from build123d import *

# Parameters (mm, degrees)
BASPROSKE_W         = 16
BASPROSKE_H         = 18
TOOTHCUT_DEPTH      = 31.066592757
TEETHCUTS_COUNT     = 16
TEETHCUTS_ANGLE     = 337.5
HUBNEAONESKE_R      = 7.5
HUBNEARONE_DEPTH    = 22.0000508
BORSKE_R            = 5
BORE_DEPTH          = 38.0000508
CUT_EXTRUDE1_START  = -10
SKETCH3_R           = 7.5
CUT_EXTRUDE1_DEPTH  = 10
BOSS_EXTRUDE1_START = -10
SKETCH4_R           = 7.5
BOSS_EXTRUDE1_DEPTH = 10
SKETCH5_R           = 5
BOSS_EXTRUDE2_DEPTH = 10


with BuildPart() as part:
    # BasProSke → Base-Revolve (revolve)
    with BuildSketch(Plane(origin=(0, 0, 0), x_dir=(1, 0, 0), z_dir=(0, 1, 0)), mode=Mode.PRIVATE) as base_revolve_sk:
        with Locations((8, 9)):
            Rectangle(BASPROSKE_W, BASPROSKE_H)
    revolve(base_revolve_sk.sketch.rotate(Axis((-10, 0, 0), (1, 0, 0)), 180), axis=Axis((-10, 0, 0), (1, 0, 0)))

    # TooCutSke → ToothCut (cut, through all)
    with BuildSketch(Plane(origin=(0, 0, 0), x_dir=(0, 0, -1), z_dir=(1, 0, 0))):
        with BuildLine():
            ThreePointArc((1.03434411, 13.459313997), (0, 13.499), (-1.03434411, 13.459313997))
            ThreePointArc((-1.03434411, 13.459313997), (-1.635143665, 15.806872195), (-3.065655864, 17.762792553))
            ThreePointArc((-3.065655864, 17.762792553), (0, 18.0254), (3.065655864, 17.762792553))
            ThreePointArc((3.065655864, 17.762792553), (1.635143665, 15.806872195), (1.03434411, 13.459313997))
        make_face()
    toothcut = extrude(amount=TOOTHCUT_DEPTH, mode=Mode.SUBTRACT)

    # TeethCuts: ToothCut ×16 about axis
    teethcuts_axis = Axis((-10, 0, 0), (1, 0, 0))
    for i in range(1, TEETHCUTS_COUNT):
        add(toothcut.rotate(teethcuts_axis, i * TEETHCUTS_ANGLE / (TEETHCUTS_COUNT - 1)), mode=Mode.SUBTRACT)

    # HubNeaOneSke → HubNearOne (add)
    with BuildSketch(Plane.ZY):
        with Locations(Location((0, 0, 0), (0, 0, 180))):
            Circle(HUBNEAONESKE_R)
    extrude(amount=HUBNEARONE_DEPTH)

    # BorSke → Bore (cut, symmetric)
    with BuildSketch(Plane(origin=(0, 0, 0), x_dir=(0, 0, -1), z_dir=(1, 0, 0))):
        with Locations(Location((0, 0, 0), (0, 0, 180))):
            Circle(BORSKE_R)
    extrude(amount=BORE_DEPTH, both=True, mode=Mode.SUBTRACT)

    # Sketch3 → Cut-Extrude1 (cut)
    with BuildSketch(Plane.ZY.offset(22.0000508).offset(CUT_EXTRUDE1_START)):
        with Locations(Location((0, 0, 0), (0, 0, 180))):
            Circle(SKETCH3_R)
    extrude(amount=CUT_EXTRUDE1_DEPTH, mode=Mode.SUBTRACT)

    # Sketch4 → Boss-Extrude1 (add)
    with BuildSketch(Plane.ZY.offset(12.0000508).offset(BOSS_EXTRUDE1_START)):
        with Locations(Location((0, 0, 0), (0, 0, 180))):
            Circle(SKETCH4_R)
    extrude(amount=BOSS_EXTRUDE1_DEPTH)

    # Sketch5 → Boss-Extrude2 (add)
    with BuildSketch(Plane.ZY.offset(12.0000508)):
        Circle(SKETCH5_R)
    extrude(amount=BOSS_EXTRUDE2_DEPTH)


solid = part.part
Source: CAD feature listing. Evaluate the final solid. Frame: model axes, mm. A direction names the side the tool comes from. Give positions to 0.01 mm unless a question says otherwise; leave off trailing zeros. Write each loop counter-clockwise with the first axis right and the second up, starting at its lowest first coordinate (ties: lowest second). Pieces come first, ordered by that corner, then holes. Notation, with made-up numbers: M 85,73 L 129,73 A19 cw 129,98 Z; hole C 22.5,65 d1. An arc over 180 degrees is marked long. Answer as a JSON object with one key per item and string values.
Q1. Ray query, line 1 along X through (y, z) = (15.5, 2); line 2 along X through (y, z) = (7, -2); line 3 along Y through (x, z) = (6.5, -1). Return the intervals inside material, ascending.
Geometry check:
{"line 1": "x = 0 to 16", "line 2": "x = -12 to 16", "line 3": "y = -13.46 to -4.9, 4.9 to 13.46"}
Q2. Access query for faces 4 (the face through (7.888, 1.614, -15.762)), 5 (the face through (7.89, 15.82, -1.64)), 6 (the face through (7.89, 9.56, 9.53)). Directions: +Z, -Z, +X, -X, +Y, -Y. A direction counts if a zero-diameter tool reaches every point of the face in a straight line with its end or side. Return the directions, or none.
Geometry check:
{"face 4": "-Z, +X, -X", "face 5": "+X, -X, +Y", "face 6": "+X, -X"}
Q3. Contact query for flat-ended pins moving along their axis: P1, Ø5, axis at x = 1.5, z = 12.5, coming from the -Y side; P2, Ø10, axis at x = -5.5, z = -11, coming from the -Y side; P3, Ø2, axis at x = -0.5, y = 5.5, coming from the +Z side. Output: stop coordinate, or through.
Geometry check:
{"P1": "stops at y = -14.97", "P2": "stops at y = -4.5", "P3": "stops at z = 12.68"}
Q4. Cut plane C-C, the plane x = -5. Return the cut outline in (y, z).
Geometry check:
{"outline": "C 0,0 d15"}
Q5. Mould query, pull axis Z, two halves, no side actions, for faces 1 (the face through (7.89, -15.82, 1.64)), 2 (the face through (7.89, -1.64, -15.82)), 3 (the face through (-16.93, -4.88, -1.08)). Classes: +Z half, -Z half, draft (parallel to the pull), parting line (faces both ways), or undercut.
Geometry check:
{"face 1": "undercut", "face 2": "-Z half", "face 3": "parting line"}
Q6. Cut plane A-A, the plane z = 0. Return the cut outline in (x, y), then the cut area to 3 significant figures.
Geometry check:
{"outline": "M -22,-5 L -12,-5 L -12,-7.5 L 0,-7.5 L 0,-13.5 L 16,-13.5 L 16,-5 L -2,-5 L -2,5 L 16,5 L 16,13.5 L 0,13.5 L 0,7.5 L -12,7.5 L -12,5 L -22,5 Z", "area": "532 mm^2"}
Q7. Cut plane D-D, the plane x = -15. Return the cut outline in (y, z).
Geometry check:
{"outline": "C 0,0 d10"}
